Autodesk Fusion 360 part; units mm, degrees
sketch "Sketch1" plane through (0, 0, 0) normal (0, 0, 1) x (1, 0, 0)
  line L0 (-7.5, 6.35) -> (7.5, 6.35)
  line L1 (7.5, 6.35) -> (7.5, 11.35)
  line L2 (7.5, 11.35) -> (-7.5, 11.35)
  line L3 (-7.5, 11.35) -> (-7.5, 6.35)
  line L4 (-7.5, 6.35) -> (7.5, 11.35) construction
  line L5 (7.5, 6.35) -> (-7.5, 11.35) construction
  line L6 (-7.5, -6.35) -> (7.5, -6.35)
  line L7 (7.5, -6.35) -> (7.5, -11.35)
  line L8 (7.5, -11.35) -> (-7.5, -11.35)
  line L9 (-7.5, -11.35) -> (-7.5, -6.35)
  line L10 (-7.5, -6.35) -> (7.5, -11.35) construction
  line L11 (7.5, -6.35) -> (-7.5, -11.35) construction
  arc A0 (-7.5, -6.35) -> (-7.5, 6.35) centre (-15.5, 0) ccw
  arc A1 (-6.2573, -6.35) -> (-6.2573, 6.35) centre (-15.5, 0) ccw
  arc A2 (7.5, 6.35) -> (7.5, -6.35) centre (15.5, 0) ccw
  arc A3 (6.2573, 6.35) -> (6.2573, -6.35) centre (15.5, 0) ccw
  circle A4 centre (-5, -8.85) radius 1
  circle A5 centre (5, -8.85) radius 1
  line L12 (-2.75, 6.35) -> (2.75, 6.35)
  line L13 (2.75, 6.35) -> (2.75, 7.35)
  line L14 (2.75, 7.35) -> (-2.75, 7.35)
  line L15 (-2.75, 7.35) -> (-2.75, 6.35)
  line L16 (-2.75, 6.35) -> (2.75, 7.35) construction
  line L17 (2.75, 6.35) -> (-2.75, 7.35) construction
  line L18 (-2.5, -6.35) -> (2.5, -6.35)
  line L19 (2.5, -6.35) -> (2.5, -7.35)
  line L20 (2.5, -7.35) -> (-2.5, -7.35)
  line L21 (-2.5, -7.35) -> (-2.5, -6.35)
  line L22 (-2.5, -6.35) -> (2.5, -7.35) construction
  line L23 (2.5, -6.35) -> (-2.5, -7.35) construction
  line L24 (0, 0) -> (-9.3045, 0) construction
  circle A6 centre (-5, 8.85) radius 1
  circle A7 centre (5, 8.85) radius 1
  point P0 (0, 8.85)
  point P1 (0, -8.85)
  point P2 (0, 6.85)
  point P3 (0, -6.85)
  dimension "d3" = 15
  dimension "d4" = 5
  dimension "d5" = 6.35
  dimension "d6" = 6.35
  dimension "d8" = 1
  dimension "d13" = 1
  dimension "d14" = 8
  dimension "d15" = 8
  dimension "d16" = 2
  dimension "d17" = 5
  dimension "d18" = 5
  dimension "d19" = 5.5
  dimension "d20" = 1
  dimension "d21" = 1
  dimension "d22" = 5
extrude "Extrude1" add sketch "Sketch1" along normal blind 3.175 contours L0 L1 L2 L3 L13 L14 L15 | L0 L6 A0 A1 | L6 L7 L8 L9 L19 L20 L21 | L0 L6 A2 A3
fillet "Fillet1" radius 0.5 8 edges at (-2.5, -7.35, 1.5875) (-2.5, -6.35, 1.5875) (-2.75, 6.35, 1.5875) (-2.75, 7.35, 1.5875) (2.75, 6.35, 1.5875) (2.75, 7.35, 1.5875) (2.5, -6.35, 1.5875) (2.5, -7.35, 1.5875)
sketch "Sketch3" plane through (0, 0, 3.175) normal (0, 0, 1) x (-1, 0, 0)
  circle A0 centre (-5, -8.85) radius 1
  circle A1 centre (5, -8.85) radius 1
  circle A2 centre (5, 8.85) radius 1
  arc A3 (-3, 6.35) -> (-2.5, 6.85) centre (-3, 6.85) ccw
  arc A4 (-2, 7.35) -> (-2.5, 6.85) centre (-2, 6.85) ccw
  line L0 (-2, 7.35) -> (2, 7.35)
  arc A5 (2.5, 6.85) -> (2, 7.35) centre (2, 6.85) ccw
  arc A6 (2.5, 6.85) -> (3, 6.35) centre (3, 6.85) ccw
  line L1 (3, 6.35) -> (6.2573, 6.35)
  arc A7 (6.2573, 6.35) -> (6.2573, -6.35) centre (15.5, 0) ccw
  line L2 (6.2573, -6.35) -> (3.25, -6.35)
  arc A8 (3.25, -6.35) -> (2.75, -6.85) centre (3.25, -6.85) ccw
  arc A9 (2.25, -7.35) -> (2.75, -6.85) centre (2.25, -6.85) ccw
  line L3 (2.25, -7.35) -> (-2.25, -7.35)
  arc A10 (-2.75, -6.85) -> (-2.25, -7.35) centre (-2.25, -6.85) ccw
  arc A11 (-2.75, -6.85) -> (-3.25, -6.35) centre (-3.25, -6.85) ccw
  line L4 (-3.25, -6.35) -> (-6.2573, -6.35)
  arc A12 (-6.2573, -6.35) -> (-6.2573, 6.35) centre (-15.5, 0) ccw
  line L5 (-6.2573, 6.35) -> (-3, 6.35)
  circle A13 centre (-5, 8.85) radius 1
  line L6 (-7.5, -11.35) -> (7.5, -11.35)
  line L7 (7.5, -11.35) -> (7.5, -6.35)
  arc A14 (7.5, 6.35) -> (7.5, -6.35) centre (15.5, 0) ccw
  line L8 (7.5, 6.35) -> (7.5, 11.35)
  line L9 (7.5, 11.35) -> (-7.5, 11.35)
  line L10 (-7.5, 11.35) -> (-7.5, 6.35)
  arc A15 (-7.5, -6.35) -> (-7.5, 6.35) centre (-15.5, 0) ccw
  line L11 (-7.5, -6.35) -> (-7.5, -11.35)
  circle A16 centre (5, 8.85) radius 1
equation "d6 = d5"
equation "d8 = d13"
equation "d11 = 0'- 1/8\""
equation "d15 = d14"
equation "d18 = d17"
equation "d21 = d20"
Can you work these out from the model? Positions are in its coordinate system, mm. A direction names the side the tool comes from. Give positions to 0.01 mm unless a question says otherwise; leave off trailing zeros. Order: outer loops, then holes, each group sorted by start corner. A loop starts at its lowest first (then second) coordinate and runs counter-clockwise, first axis right, second up. Notation, with made-up numbers: M 58.5,77 L 101.5,77 A26 cw 101.5,102 Z; hole C -5,37 d9. An arc over 180 degrees is marked long. Write item = value, one per line. Start each with the question number.
Q1. Suppose I cut it at C-C (x = 0.5). Write out the boundary of the cut face in (y, z) (3 decimals), plus the area to 3 significant figures.
Q2. Suppose I cut it at A-A (y = 8.85). Write out the boundary of the cut face in (x, z) (3 decimals), plus the area to 3 significant figures.
Q3. We'd pull the mould along X, two halves only. Please class faces 1 (the cylindrical face through (-5.217, -7.874, 1.565)), 2 (the flat face through (-7.5, -9, 2)), 3 (the cylindrical face through (4.783, -7.874, 1.565)), 4 (the flat face through (7.5, -9, 2)): pulls with the +X half, pulls with the -X half, needs draft (parallel to the pull), parting line crosses it, or undercut.
Q4. Suppose I cut it at B-B (z = 2.4). Count the separate pieces of the cut face and the enclosed holes in it, plus the area to 3 significant figures.
Q5. Suppose I cut it at D-D (y = 0.5). Write out the boundary of the cut face in (x, z) (3 decimals).
Q6. For faces 5 (the cylindrical face through (5.287, -0.096, 1.565)), 6 (the flat face through (0, 7.35, 2)), which set-ups out of +Z, -Z, +X, -X, +Y, -Y let a thin tool reach every point of the face, with its end or its side?
Q7. I need wall thicknesses on probe 1 along Y at (x, z) = (-0.5, 0.45); probe 2 along Y at (x, z) = (4.25, 1.95); probe 3 along X at (y, z) = (9.5, 2.9). Which ranges of each line are inside material? Lowest first, please. Write a range as [from, to].
Q8. Will this pin go through, and if not, where does the flat tip stop? pin 1 Ø1 at (y, z) = (-0.5, 2) entering from +X.
Check result:
q1.outline = M -11.35,0 L -7.35,0 L -7.35,3.175 L -11.35,3.175 Z; M 7.35,0 L 11.35,0 L 11.35,3.175 L 7.35,3.175 Z
q1.area = 25.4 mm2
q2.outline = M -7.5,0 L -6,0 L -6,3.175 L -7.5,3.175 Z; M -4,0 L 4,0 L 4,3.175 L -4,3.175 Z; M 6,0 L 7.5,0 L 7.5,3.175 L 6,3.175 Z
q2.area = 34.9 mm2
q3.face_1 = undercut
q3.face_2 = pulls with the -X half
q3.face_3 = undercut
q3.face_4 = pulls with the +X half
q4.separate_pieces = 1
q4.enclosed_holes = 5
q4.area = 154 mm2
q5.outline = M -5.298,0 L -4.297,0 L -4.297,3.175 L -5.298,3.175 Z; M 4.297,0 L 5.298,0 L 5.298,3.175 L 4.297,3.175 Z
q6.face_5 = +Z, -Z, +X
q6.face_6 = +Z, -Z
q7.probe_1 = [-11.35, -7.35], [7.35, 11.35]
q7.probe_2 = [-11.35, -9.51], [-8.19, -6.35], [6.35, 8.19], [9.51, 11.35]
q7.probe_3 = [-7.5, -5.76], [-4.24, 4.24], [5.76, 7.5]
q8.pin_1 = 5.34
